Geometry: final body of the model. Coordinates: model frame, mm. A direction names the side the tool comes from. Give positions to 0.01 mm unless a question says otherwise; leave off trailing zeros. Order: outer loops, then holes, each group sorted by start corner. A loop starts at its lowest first (then second) coordinate and runs counter-clockwise, first axis right, second up. Notation, with made-up numbers: (24.25, -26) -> (40.25, -26) arc R15 ccw to (40.25, -15) -> close; hole circle Ø1 at (-0.5, 73.25). An arc over 180 degrees is marked (long way). Write item = value, one per line.
```python
from build123d import *

# Parameters (mm, degrees)
SKETCH1_R                   = 20
BOSS_EXTRUDE1_DEPTH         = 35
SKETCH3_R                   = 10
BOSS_EXTRUDE3_DEPTH         = 5
SKETCH4_R                   = 7.5
CUT_EXTRUDE1_DEPTH          = 1
SKETCH5_R                   = 3
BOSS_EXTRUDE4_DEPTH         = 14
SKETCH6_W                   = 5.83666228
SKETCH6_H                   = 4.189609368
CUT_EXTRUDE2_DEPTH          = 10
TAP_DRILL_FOR_M3_TAP1_D     = 2.5
TAP_DRILL_FOR_M3_TAP1_DEPTH = 8
TAP_DRILL_FOR_M3_TAP1_TIP   = 0.751075774
SKETCH10_W                  = 2.171108564
SKETCH10_H                  = 0.2
SKETCH11_R                  = 3.5
BOSS_EXTRUDE5_DEPTH         = 21
SKETCH12_R                  = 2
FILLET1_R                   = 2


with BuildPart() as part:
    # Sketch1 → Boss-Extrude1 (new body)
    with BuildSketch(Plane(origin=(0, 0, 0), x_dir=(1, 0, 0), z_dir=(0, 1, 0))):
        with Locations(Location((0, 0, 0), (0, 0, 270))):
            Circle(SKETCH1_R)
    extrude(amount=BOSS_EXTRUDE1_DEPTH)

    # Sketch3 → Boss-Extrude3 (add)
    with BuildSketch(Plane(origin=(0, 35, 0), x_dir=(1, 0, 0), z_dir=(0, 1, 0))):
        with Locations(Location((0, 0, 0), (0, 0, 270))):
            Circle(SKETCH3_R)
    extrude(amount=BOSS_EXTRUDE3_DEPTH)

    # Sketch4 → Cut-Extrude1 (cut)
    with BuildSketch(Plane(origin=(0, 40, 0), x_dir=(1, 0, 0), z_dir=(0, 1, 0))):
        with Locations(Location((0, 0, 0), (0, 0, 270))):
            Circle(SKETCH4_R)
    extrude(amount=-CUT_EXTRUDE1_DEPTH, mode=Mode.SUBTRACT)

    # Sketch5 → Boss-Extrude4 (add)
    with BuildSketch(Plane(origin=(0, 39, 0), x_dir=(1, 0, 0), z_dir=(0, 1, 0))):
        with Locations(Location((0, 0, 0), (0, 0, 270))):
            Circle(SKETCH5_R)
    extrude(amount=BOSS_EXTRUDE4_DEPTH)

    # Sketch6 → Cut-Extrude2 (cut)
    with BuildSketch(Plane(origin=(0, 53, 0), x_dir=(1, 0, 0), z_dir=(0, 1, 0))):
        with Locations((0, 4.594804684)):
            Rectangle(SKETCH6_W, SKETCH6_H)
    extrude(amount=-CUT_EXTRUDE2_DEPTH, mode=Mode.SUBTRACT)

    # Tap Drill for M3 Tap1
    with Locations(Plane(origin=(0, 35, 0), x_dir=(1, 0, 0), z_dir=(0, 1, 0))):
        with Locations((0, 14), (7.5, 12.990381057), (7.5, -12.990381057), (12.124355653, -7), (-12.124355653, -7), (-15, 0)):
            Hole(TAP_DRILL_FOR_M3_TAP1_D / 2, depth=TAP_DRILL_FOR_M3_TAP1_DEPTH)
            with Locations((0, 0, -(TAP_DRILL_FOR_M3_TAP1_DEPTH + TAP_DRILL_FOR_M3_TAP1_TIP / 2))):  # 118° drill point
                Cone(0, TAP_DRILL_FOR_M3_TAP1_D / 2, TAP_DRILL_FOR_M3_TAP1_TIP, mode=Mode.SUBTRACT)

    # Sketch10 → Cut-Revolve1 (revolve, cut)
    with BuildSketch(Plane.XY, mode=Mode.PRIVATE) as cut_revolve1_sk:
        with Locations((20, 31.9)):
            Rectangle(SKETCH10_W, SKETCH10_H)
    revolve(cut_revolve1_sk.sketch.rotate(Axis((0, 0, 0), (0, 1, 0)), 123.557309762), axis=Axis((0, 0, 0), (0, 1, 0)), mode=Mode.SUBTRACT)

    # Sketch11 → Boss-Extrude5 (add)
    with BuildSketch(Plane.XY):
        with Locations(Location((0, 7.305759765, 0), (0, 0, 180))):
            Circle(SKETCH11_R)
    extrude(amount=BOSS_EXTRUDE5_DEPTH)

    # Sweep1: sweep along a path in Sketch13
    with BuildLine() as sweep1_path:  # in the path sketch's own coordinates; laid on its plane below (add() does not lay a ready-made edge on the line's plane)
        add(Edge.make_bspline(
            [(-21, 7.305759765), (-39.680829044, 7.305759765), (-58.658536918, -3.239081936), (-76.270922844, 9.376545434)],
            knots=[0, 0, 0, 0, 1, 1, 1, 1], degree=3))
    # Sketch12 → Sweep1 (sweep)
    with BuildSketch(Plane.XY.offset(21)):
        with Locations((0, 7.305759765)):
            Circle(SKETCH12_R)
    sweep(path=Plane(origin=(0, 0, 0), x_dir=(0, 0, -1), z_dir=(1, 0, 0)) * sweep1_path.line)

    # Fillet1
    fillet1_edges = [part.edges().sort_by_distance(p)[0] for p in [
        (0, 0, -20),
    ]]
    fillet(fillet1_edges, radius=FILLET1_R)


solid = part.part
```
1) Section query B-B (y = 19.5). Output: boundary loops of the cut face in (x, z), plus the area to 3 significant figures.
Check sheet entries:
outline = circle Ø40 at (0, 0)
area = 1,260 mm²
2) First-contact query: P1, Ø3.5, axis at x = -0.5, y = 47, coming from the -Z side; P2, Ø4, axis at x = -11.5, y = 30, coming from the +Z side; P3, Ø10, axis at x = 7.5, z = 18.5, coming from the +Y side. Flat tips, straight axial feed; report the tip coordinate or a pass-through.
Check sheet entries:
P1 = -2.5
P2 = 17.6
P3 = 35
3) Reachability of faces 4 (the face through (9, 35, -5)), 5 (the face through (2.1, 8.1, 21)) from +Z, -Z, +X, -X, +Y, -Y: full face, straight path, thin tool, end or side. Return the list, or none.
Check sheet entries:
face_4 = +Y
face_5 = none
4) Section query D-D (y = 50). Output: boundary loops of the cut face in (x, z), plus the area to 3 significant figures.
Check sheet entries:
outline = (-1.66, -2.5) -> (1.66, -2.5) arc R3 ccw (long way) to start
area = 27.1 mm²
5) Mould query, pull axis Z, two halves, no side actions, for faces 1 (the face through (0, 53, 0)), 2 (the face through (0.16, 30.94, -15.24)), 3 (the face through (-0.1, 9.362, 76.281)). Classes: +Z half, -Z half, draft (parallel to the pull), parting line (faces both ways), or undercut.
Check sheet entries:
face_1 = draft
face_2 = undercut
face_3 = +Z half
6) Section query A-A (y = 28). Output: boundary loops of the cut face in (x, z), plus the area to 3 significant figures.
Check sheet entries:
outline = circle Ø40 at (0, 0); hole circle Ø2.5 at (-15, 0); hole circle Ø2.5 at (-12.12, 7); hole circle Ø2.5 at (0, -14); hole circle Ø2.5 at (7.5, -12.99); hole circle Ø2.5 at (7.5, 12.99); hole circle Ø2.5 at (12.12, 7)
area = 1,230 mm²
7) Section query C-C (y = 37). Output: boundary loops of the cut face in (x, z).
Check sheet entries:
outline = circle Ø20 at (0, 0)
8) Line query: line 1 (Y direction, x = 5.5, z = -3.5); line 2 (Y direction, x = -3, z = -7); line 3 (Z direction, x = -15, y = 28.5). Output: solid intervals per line, ascending. Write a range as from..to.
Check sheet entries:
line_1 = 0..39
line_2 = 0..40
line_3 = -13.23..-1.25, 1.25..13.23
